Can you work these out from the drawing? Everything is in mm from the part's minimum corner. A direction names the side the tool comes from. Round coordinates to 2 decimals unless told otherwise and drop trailing zeros. Loops run counter-clockwise (first coordinate to the right, second up) from the corner with the lowest first, then second, coordinate; pieces in that order, holes last. Notation, with made-up numbers: (67.25, 57.25) -> (76.25, 57.25) arc R10 ccw to (76.25, 72.25) -> close; hole circle Ø5 at (42, 49.25). An arc over 180 degrees is marked (long way). One line per item, written item: value.
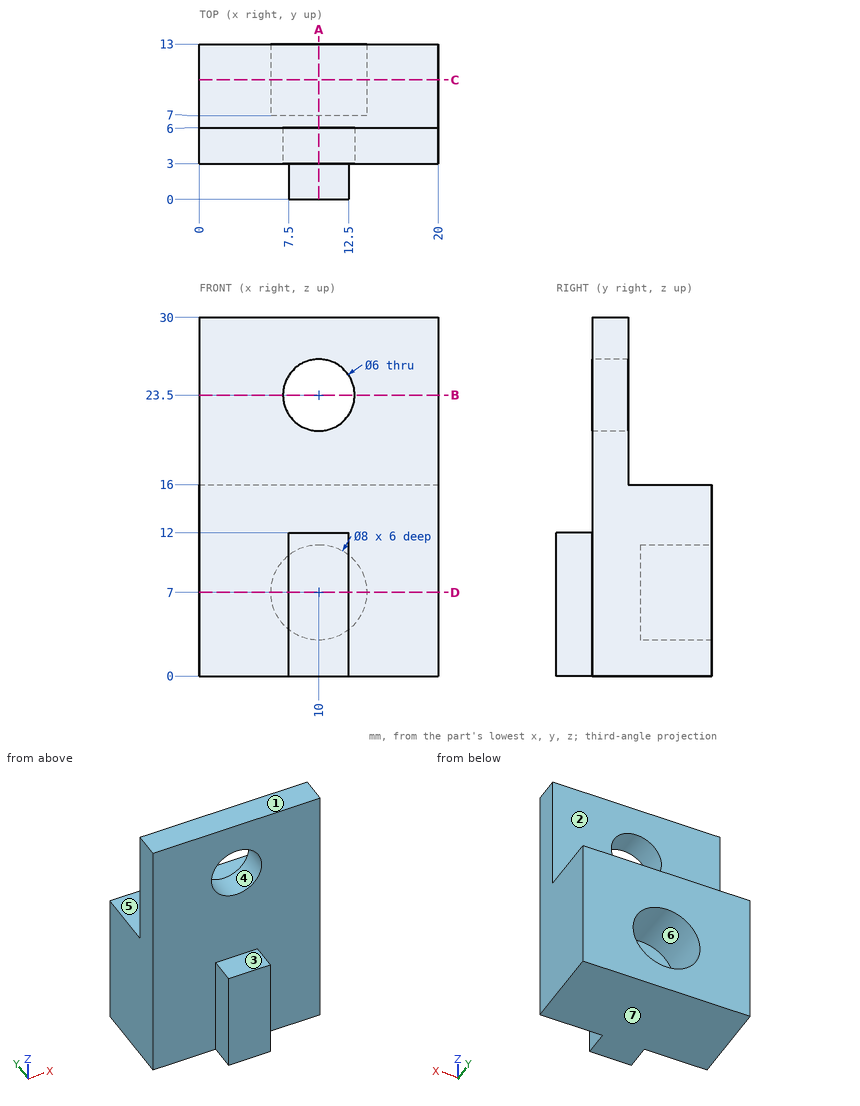
(1) For pin 1 Ø1 at (x, z) = (15.5, 16.5) entering from -Y; pin 2 Ø11 at (x, z) = (5.5, 26) entering from +Y; pin 3 Ø2 at (x, y) = (14, 10) entering from +Z, each with a flat end and sliding along its axis, tell me the tip position at first contact or that it passes through.
Results below:
pin 1: stops at y = 3
pin 2: stops at y = 6
pin 3: stops at z = 16
(2) Imagine slicing it at C-C on y = 10. Write out the boundary of the cut face in (x, z), then the cut area to 3 significant figures.
Results below:
outline: (0, 0) -> (20, 0) -> (20, 16) -> (0, 16) -> close; hole circle Ø8 at (10, 7)
area: 270 mm²
(3) Imagine slicing it at D-D on z = 7. Write out the boundary of the cut face in (x, y), then the cut area to 3 significant figures.
Results below:
outline: (0, 3) -> (7.5, 3) -> (7.5, 0) -> (12.5, 0) -> (12.5, 3) -> (20, 3) -> (20, 13) -> (14, 13) -> (14, 7) -> (6, 7) -> (6, 13) -> (0, 13) -> close
area: 167 mm²
(4) Imagine slicing it at B-B on z = 23.5. Write out the boundary of the cut face in (x, y), then the cut area to 3 significant figures.
Results below:
outline: (0, 3) -> (7, 3) -> (7, 6) -> (0, 6) -> close; (13, 3) -> (20, 3) -> (20, 6) -> (13, 6) -> close
area: 42.0 mm²
(5) Imagine slicing it at A-A on x = 10. Write out the boundary of the cut face in (y, z).
Results below:
outline: (0, 0) -> (13, 0) -> (13, 3) -> (7, 3) -> (7, 11) -> (13, 11) -> (13, 16) -> (6, 16) -> (6, 20.5) -> (3, 20.5) -> (3, 12) -> (0, 12) -> close; (3, 26.5) -> (6, 26.5) -> (6, 30) -> (3, 30) -> close
(6) Please list where these lines run through material, in increasing order: L1, parallel to X at y = 4.3, z = 23.5; L2, parallel to X at y = 8.95, z = 7; L3, parallel to Z at x = 11.75, y = 1.5.
Results below:
L1: x = 0 to 7, 13 to 20
L2: x = 0 to 6, 14 to 20
L3: z = 0 to 12
(7) We'd pull the mould along Z, two halves only. Please class the marked faces 4, 5, 6 and 7: +Z half, -Z half, draft (parallel to the pull), parting line (faces both ways), or undercut.
Results below:
face 4: undercut
face 5: +Z half
face 6: undercut
face 7: -Z half
(8) On a 3-axis mill with a long thin cutter (end or side, diameter ignored), from which of +Z, -Z, +X, -X, +Y, -Y can I reach the whole of each face in a straight line? I mean the marked faces 1, 2 and 3. Say none if no direction works.
Results below:
face 1: +Z, +X, -X, +Y, -Y
face 2: +Z, +X, -X, +Y
face 3: +Z, +X, -X, -Y
